Source: CAD feature listing. Evaluate the final solid. Frame: model axes, mm. Face numbers are marked on the shaded views. A direction names the side the tool comes from. Coordinates: 2 decimals unless noted, no trailing zeros. Write each loop counter-clockwise with the first axis right and the second up, starting at its lowest first coordinate (ties: lowest second). Pieces come first, ordered by that corner, then holes. Notation, with made-up numbers: (-36.75, 61) - (14.25, 61) arc R30 cw to (14.25, 84) - close; hole circle Ø1 at (-11.5, 46.5). An arc over 180 degrees is marked (long way). One line per item, written item: value.
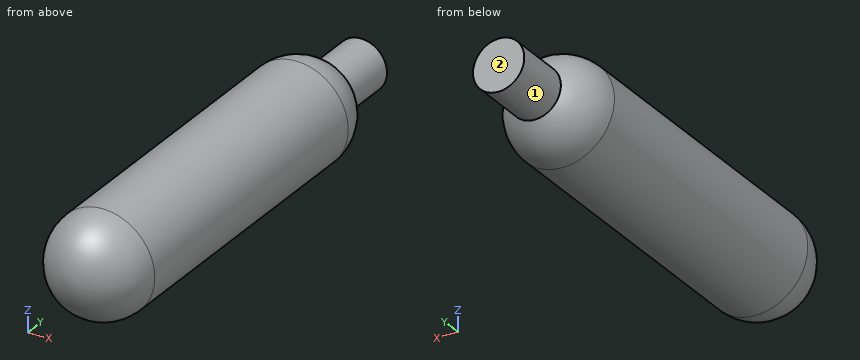
from build123d import *

# Parameters (mm, degrees)
F0_R     = 6.35
F1_DEPTH = 50.8
F2_R     = 6.35
F3_R     = 6.35
F4_R     = 3.175
F5_DEPTH = 6.35


with BuildPart() as f1:
    # F0 (on Front) → F1 (new body)
    with BuildSketch(Plane.XZ):
        Circle(F0_R)
    extrude(amount=F1_DEPTH)

    # F2
    f2_edges = [f1.edges().sort_by_distance(p)[0] for p in [
        (-6.35, -50.8, 0),
    ]]
    fillet(f2_edges, radius=F2_R)

    # F3
    f3_edges = [f1.edges().sort_by_distance(p)[0] for p in [
        (-6.35, 0, 0),
    ]]
    fillet(f3_edges, radius=F3_R)

    # F4 (on Front) → F5 (join, symmetric)
    with BuildSketch(Plane.XZ):
        Circle(F4_R)
    extrude(amount=F5_DEPTH, both=True)


solid = f1.part
1) Reachability of the marked faces 1 and 2 from +Z, -Z, +X, -X, +Y, -Y: full face, straight path, thin tool, end or side. Return the list, or none.
Values found:
face 1: +Y
face 2: +Z, -Z, +X, -X, +Y
2) Section query C-C on y = -17. Output: boundary loops of the cut face in (x, z).
Values found:
outline: circle Ø12.7 at (0, 0)
3) Section query B-B on x = 0. Output: boundary loops of the cut face in (y, z) (3 decimals).
Values found:
outline: (-44.45, -6.35) - (-6.35, -6.35) arc R6.35 ccw to (-0.851, -3.175) - (6.35, -3.175) - (6.35, 3.175) - (-0.851, 3.175) arc R6.35 ccw to (-6.35, 6.35) - (-44.45, 6.35) arc R6.35 ccw to start
4) Material intervals for line 1 (Z direction, x = -5.5, y = -18); line 2 (Z direction, x = -2.5, y = 3); line 3 (Y direction, x = -3.75, z = -1.5), sorted ascending.
Values found:
line 1: -3.17 to 3.17
line 2: -1.96 to 1.96
line 3: -49.35 to -1.45
5) Contact query for flat-ended pins moving along their axis: P1, Ø1.5, axis at x = 1, z = -1.5, coming from the -Y side; P2, Ø1, axis at x = -1.5, y = -44, coming from the +Z side; P3, Ø2, axis at x = -0.5, z = 2.5, coming from the -Y side; P4, Ø4, axis at y = -13.5, z = -1, coming from the +X side. Output: stop coordinate, or through.
Values found:
P1: y = -50.71
P2: z = 6.27
P3: y = -50.61
P4: x = 6.35
6) Section query D-D on y = 3.5. Output: boundary loops of the cut face in (x, z) (3 decimals).
Values found:
outline: circle Ø6.35 at (0, 0)
7) Section query A-A on z = 0. Output: boundary loops of the cut face in (x, y) (3 decimals).
Values found:
outline: (-6.35, -44.45) arc R6.35 ccw to (6.35, -44.45) - (6.35, -6.35) arc R6.35 ccw to (3.175, -0.851) - (3.175, 6.35) - (-3.175, 6.35) - (-3.175, -0.851) arc R6.35 ccw to (-6.35, -6.35) - close
